Work out the finished part from the listing and answer in its coordinate system (mm). A direction names the side the tool comes from. Coordinates: 2 decimals unless noted, no trailing zeros. Loops run counter-clockwise (first coordinate to the right, second up) from the corner with the lowest first, then second, coordinate; pieces in that order, holes last. Notation, with made-up numbers: (27.25, 5.5) -> (73.25, 5.5) arc R22 cw to (73.25, 30.5) -> close; hole circle Ø11 at (61.25, 3.5). An arc over 180 degrees is marked (long way). Use a Markdown table: item, result.
from build123d import *

# Parameters (mm, degrees)
F1_DEPTH = 25
F2_R     = 1.5
F3_R     = 2.5
F4_DEPTH = 25


with BuildPart() as f1:
    # F0 (on Front) → F1 (new body)
    with BuildSketch(Plane.XZ):
        Polygon((10, 3.1115), (10, 10), (3.1115, 10), (3.1115, 8.222), (5.461, 8.222), (5.461, 6.444), (3.1115, 3.777), (0, 3.777), (-3.1115, 3.777), (-5.461, 6.444), (-5.461, 8.222), (-3.1115, 8.222), (-3.1115, 10), (-10, 10), (-10, 3.1115), (-8.222, 3.1115), (-8.222, 5.461), (-6.444, 5.461), (-3.777, 3.1115), (-3.777, 0), (-3.777, -3.1115), (-6.444, -5.461), (-8.222, -5.461), (-8.222, -3.1115), (-10, -3.1115), (-10, -10), (-3.1115, -10), (-3.1115, -8.222), (-5.461, -8.222), (-5.461, -6.444), (-3.1115, -3.777), (0, -3.777), (3.1115, -3.777), (5.461, -6.444), (5.461, -8.222), (3.1115, -8.222), (3.1115, -10), (10, -10), (10, -3.1115), (8.222, -3.1115), (8.222, -5.461), (6.444, -5.461), (3.777, -3.1115), (3.777, 0), (3.777, 3.1115), (6.444, 5.461), (8.222, 5.461), (8.222, 3.1115), align=None)
    extrude(amount=F1_DEPTH)

    # F2
    f2_edges = [f1.edges().sort_by_distance(p)[0] for p in [
        (-10, -12.5, 10),
        (10, -12.5, 10),
        (10, -12.5, -10),
        (-10, -12.5, -10),
    ]]
    fillet(f2_edges, radius=F2_R)

    # F3 (on face) → F4 (cut, through all)
    with BuildSketch(Plane.XZ.offset(25)):
        Circle(F3_R)
    extrude(amount=-F4_DEPTH, mode=Mode.SUBTRACT)


solid = f1.part
Q1. Section A-A on x = 6.75 is taken. Determine the outline of the cut face in (y, z).
Solved:
| item | result |
|---|---|
| outline | (-25, -10) -> (0, -10) -> (0, -5.46) -> (-25, -5.46) -> close; (-25, 5.46) -> (0, 5.46) -> (0, 10) -> (-25, 10) -> close |
Q2. Section C-C on z = 5 is taken. Determine the outline of the cut face in (x, y).
Solved:
| item | result |
|---|---|
| outline | (-10, -25) -> (-8.22, -25) -> (-8.22, 0) -> (-10, 0) -> close; (-5.92, -25) -> (-4.19, -25) -> (-4.19, 0) -> (-5.92, 0) -> close; (4.19, -25) -> (5.92, -25) -> (5.92, 0) -> (4.19, 0) -> close; (8.22, -25) -> (10, -25) -> (10, 0) -> (8.22, 0) -> close |
Q3. Given pin 1 Ø2 at (x, z) = (-4.5, -7) entering from -Y; pin 2 Ø0.5 at (y, z) = (-18.5, 9) entering from +X, each flat-ended and moving along its own axis, determine where each tip first touches the part or whether it passes through.
Solved:
| item | result |
|---|---|
| pin 1 | y = -25 |
| pin 2 | x = 9.98 |
Q4. Determine the mould class of faces 6 (the cylindrical face through (9.55, -12.68, -9.57)), 7 (the flat face through (-7, -12, -5.461)), 8 (the flat face through (-10, -12, -6)), 9 (the flat face through (-4.303, -12.325, -5.129)) for opening direction Z: pulls with the +Z half, pulls with the -Z half, needs draft (parallel to the pull), parting line crosses it, or undercut.
Solved:
| item | result |
|---|---|
| face 6 | pulls with the -Z half |
| face 7 | undercut |
| face 8 | needs draft |
| face 9 | undercut |
Q5. Section B-B on z = 0 is taken. Determine the outline of the cut face in (x, y).
Solved:
| item | result |
|---|---|
| outline | (-3.78, -25) -> (-2.5, -25) -> (-2.5, 0) -> (-3.78, 0) -> close; (2.5, -25) -> (3.78, -25) -> (3.78, 0) -> (2.5, 0) -> close |
Q6. For faces 1 (the flat face through (3.112, -12, 9)), 2 (the flat face through (2, -25, 2)), 3 (the flat face through (8.222, -12, -4)), 4 (the cylindrical face through (-9.55, -12.68, 9.57)), 5 (the flat face through (0, -12, -3.777)), determine the directions among +Z, -Z, +X, -X, +Y, -Y from which every point of the face is accessible in a straight line to the end or side of a thin tool.
Solved:
| item | result |
|---|---|
| face 1 | +Z, +Y, -Y |
| face 2 | +Z, -Z, +X, -X, -Y |
| face 3 | +Y, -Y |
| face 4 | +Z, -X, +Y, -Y |
| face 5 | -Z, +Y, -Y |
Q7. Consider line 1 (Z direction, x = 0, y = -11.75); line 2 (X direction, y = -21.5, z = 8); line 3 (X direction, y = -3.75, z = -5.25). Determine where each line is inside the solid, lowest interval first. Write a range as [from, to].
Solved:
| item | result |
|---|---|
| line 1 | [-3.78, -2.5], [2.5, 3.78] |
| line 2 | [-10, -5.46], [5.46, 10] |
| line 3 | [-10, -8.22], [-6.2, -4.41], [4.41, 6.2], [8.22, 10] |
